Input: part model. Units: mm. Frame: model coordinates. A direction names the side the tool comes from. Round coordinates to 2 decimals unless told otherwise and drop trailing zeros. Loops run counter-clockwise (first coordinate to the right, second up) from the corner with the lowest first, then second, coordinate; pieces in that order, holes last. Notation, with made-up numbers: (15, 72.25) -> (26, 72.25) arc R21 ccw to (26, 100.25) -> close; hole circle Ø11 at (-11.5, 43). An arc over 180 degrees is marked (long way). One line per question, with ' | ' between items. Start each with the question number.
Q1. Mould query, pull axis Z, two halves, no side actions, for faces 4 (the face through (119, 4, -6)), 5 (the face through (106, 0, -7)), 6 (the face through (116, 4, -50)). Classes: pulls with the +Z half, pulls with the -Z half, needs draft (parallel to the pull), parting line crosses it, or undercut.
Q2. Cut plane B-B on x = 98. Return loops of the section in (y, z).
Q3. Material intervals for L1, parallel to X at y = 1.15, z = -5.5; L2, parallel to Z at x = 17, y = -1.4; L3, parallel to Z at x = 24, y = 1.6, sorted ascending.
Q4. Cut plane C-C on z = -90. State how many separate pieces and enclosed holes the cut face has, and give its area (3 significant figures).
Q5. Access query for faces 1 (the face through (20.233, -1.521, -6.841)), 2 (the face through (73, 4, -6)), 3 (the face through (77.8, 4, -50)). Directions: +Z, -Z, +X, -X, +Y, -Y. A direction counts if a zero-diameter tool reaches every point of the face in a straight line with its end or side. Return the directions, or none.
Q6. Cut plane A-A on z = -26.5. Return loops of the section in (x, y).
Q7. Contact query for flat-ended pins moving along their axis: P1, Ø4, axis at x = 24, z = -90, coming from the -Y side; P2, Ø0.9, axis at x = 48.5, y = 4.5, coming from the +Z side; P3, Ø1.5, axis at x = 60.5, z = -69.5, coming from the +Y side. Output: stop coordinate, or through.
from build123d import *

# Parameters (mm, degrees)
SKETCH1_W                   = 122
SKETCH1_H                   = 100
BOSS_EXTRUDE1_DEPTH         = 3
SKETCH2_W                   = 6
SKETCH2_H                   = 50
SKETCH2_W_2                 = 11
SKETCH2_H_2                 = 90
SKETCH2_H_3                 = 25
BOSS_EXTRUDE2_DEPTH         = 3
SKETCH3_W                   = 3
SKETCH3_H                   = 40
BOSS_EXTRUDE3_DEPTH         = 1.5
SKETCH4_W                   = 122
SKETCH4_H                   = 4
BOSS_EXTRUDE4_DEPTH         = 3
SKETCH7_W                   = 122
SKETCH7_H                   = 100
BOSS_EXTRUDE5_DEPTH         = 3
SKETCH5_R                   = 1.6
STANDOFF_HOLE_DEPTH         = 4
STANDOFF_HOLE_DEPTH_BACK    = 7
SKETCH6_R                   = 3.5
CLEARANCE_HOLE_TOP_DEPTH    = 4
SKETCH8_R                   = 3.5
CLEARANCE_HOLE_BOTTOM_DEPTH = 3


with BuildPart() as part:
    # Sketch1 → Boss-Extrude1 (new body)
    with BuildSketch(Plane(origin=(0, 0, 0), x_dir=(1, 0, 0), z_dir=(0, 1, 0))):
        with Locations((61, 50)):
            Rectangle(SKETCH1_W, SKETCH1_H)
    extrude(amount=BOSS_EXTRUDE1_DEPTH)

    # Sketch2 → Boss-Extrude2 (add)
    with BuildSketch(Plane(origin=(0, 3, 0), x_dir=(1, 0, 0), z_dir=(0, 1, 0))):
        with Locations((3, 71)):
            Rectangle(SKETCH2_W, SKETCH2_H)
        with Locations((13.8, 51)):
            Rectangle(SKETCH2_W_2, SKETCH2_H_2)
        with Locations((38.8, 51)):
            Rectangle(SKETCH2_W_2, SKETCH2_H_2)
        with Locations((49.3, 71)):
            Rectangle(SKETCH2_W, SKETCH2_H)
        with Locations((72.8, 18.5)):
            Rectangle(SKETCH2_W, SKETCH2_H_3)
        with Locations((83.3, 51)):
            Rectangle(SKETCH2_W_2, SKETCH2_H_2)
        with Locations((108.3, 51)):
            Rectangle(SKETCH2_W_2, SKETCH2_H_2)
        with Locations((119, 51)):
            Rectangle(SKETCH2_W, SKETCH2_H_2)
    extrude(amount=BOSS_EXTRUDE2_DEPTH)

    # Sketch3 → Boss-Extrude3 (add)
    with BuildSketch(Plane(origin=(0, 3, 0), x_dir=(1, 0, 0), z_dir=(0, 1, 0))):
        with Locations((57.1, 76)):
            Rectangle(SKETCH3_W, SKETCH3_H)
    extrude(amount=BOSS_EXTRUDE3_DEPTH)

    # Sketch4 → Boss-Extrude4 (add)
    with BuildSketch(Plane(origin=(0, 3, 0), x_dir=(1, 0, 0), z_dir=(0, 1, 0))):
        with Locations((61, 98)):
            Rectangle(SKETCH4_W, SKETCH4_H)
    extrude(amount=BOSS_EXTRUDE4_DEPTH)

    # Sketch7 → Boss-Extrude5 (add)
    with BuildSketch(Plane.XZ):
        with Locations((61, -50)):
            Rectangle(SKETCH7_W, SKETCH7_H)
    extrude(amount=BOSS_EXTRUDE5_DEPTH)

    # Sketch5 → standoff hole (cut, two sides)
    with BuildSketch(Plane(origin=(0, 3, 0), x_dir=(1, 0, 0), z_dir=(0, 1, 0))) as standoff_hole_sk:
        with Locations((17, 5.5)):
            Circle(SKETCH5_R)
        with Locations((105, 5.5)):
            Circle(SKETCH5_R)
        with Locations((24, 90)):
            Circle(SKETCH5_R)
        with Locations((98, 90)):
            Circle(SKETCH5_R)
    extrude(amount=STANDOFF_HOLE_DEPTH, mode=Mode.SUBTRACT)
    extrude(standoff_hole_sk.sketch, amount=-STANDOFF_HOLE_DEPTH_BACK, mode=Mode.SUBTRACT)

    # Sketch6 → clearance hole top (cut, through all)
    with BuildSketch(Plane(origin=(0, 3, 0), x_dir=(1, 0, 0), z_dir=(0, 1, 0))):
        with Locations((17, 5.5)):
            Circle(SKETCH6_R)
        with Locations((105, 5.5)):
            Circle(SKETCH6_R)
    extrude(amount=CLEARANCE_HOLE_TOP_DEPTH, mode=Mode.SUBTRACT)

    # Sketch8 → clearance hole bottom (cut)
    with BuildSketch(Plane.XZ.offset(3)):
        with Locations((17, -5.5)):
            Circle(SKETCH8_R)
        with Locations((105, -5.5)):
            Circle(SKETCH8_R)
        with Locations((98, -90)):
            Circle(SKETCH8_R)
        with Locations((24, -90)):
            Circle(SKETCH8_R)
    extrude(amount=-CLEARANCE_HOLE_BOTTOM_DEPTH, mode=Mode.SUBTRACT)


solid = part.part
Results:
1) face 4: pulls with the +Z half | face 5: undercut | face 6: needs draft
2) outline: (-3, -100) -> (6, -100) -> (6, -96) -> (3, -96) -> (3, -91.6) -> (0, -91.6) -> (0, -93.5) -> (-3, -93.5) -> close; (-3, -86.5) -> (0, -86.5) -> (0, -88.4) -> (3, -88.4) -> (3, 0) -> (-3, 0) -> close
3) L1: 0 to 15.4, 18.6 to 103.4, 106.6 to 122 | L2: -100 to -9, -2 to 0 | L3: -100 to -91.6, -88.4 to 0
4) separate pieces: 3 | enclosed holes: 0 | area: 861 mm^2
5) face 1: -Y | face 2: +Z, +X, -X, +Y | face 3: +Z, +Y
6) outline: (0, -3) -> (122, -3) -> (122, 6) -> (116, 6) -> (116, 3) -> (113.8, 3) -> (113.8, 6) -> (102.8, 6) -> (102.8, 3) -> (88.8, 3) -> (88.8, 6) -> (77.8, 6) -> (77.8, 3) -> (75.8, 3) -> (75.8, 6) -> (69.8, 6) -> (69.8, 3) -> (44.3, 3) -> (44.3, 6) -> (33.3, 6) -> (33.3, 3) -> (19.3, 3) -> (19.3, 6) -> (8.3, 6) -> (8.3, 3) -> (0, 3) -> close
7) P1: y = 0 | P2: z = -46 | P3: y = 3
